For this review, take the finished solid that the model builds, in its own axes (mm). A direction names the side the tool comes from. Round coordinates to 2 decimals unless told otherwise and drop trailing zeros. Order: outer loops, then holes, each group sorted by start corner. A loop starts at its lowest first (then second) coordinate and runs counter-clockwise, first axis right, second up. Notation, with made-up numbers: (-27.5, 24.5) -> (-18.5, 24.5) arc R26 ccw to (-18.5, 43.5) -> close; hole circle Ø1 at (64, 47). An arc over 180 degrees is marked (long way). Use a Markdown table: item, result. Add a question column.
1) Wall thickness on line 1 along Z through (x, y) = (-2.75, -43.8); line 2 along Z through (x, y) = (-6.5, -43.8); line 3 along Z through (x, y) = (-1.75, 55): over which ranges is each line inside the solid? List them lowest first. Write a range as [from, to].
2) Machinability: for faces 5 (the face through (2, -68.8, 0)), 6 (the face through (1.5, -62.37, 16.52)), 7 (the face through (5, 70, 0)), which of the approach directions +Z, -Z, +X, -X, +Y, -Y give a long, thin tool a straight path to every point of the face, cutting with its end or side? Answer none if there is none.
3) Consider section A-A (y = 43.8). State the section outline as (x, z) points, plus the area to 4 significant figures.
4) Clearance check with flat-ended pins moving along their axes: P1, Ø6, axis at x = -3.5, z = -2, coming from the +Y side; P2, Ø6.5, axis at y = 46.5, z = -11.5, coming from the +X side; P3, Ø2, axis at y = 49, z = -1, coming from the +X side; P4, Ø11, axis at y = 43.8, z = 14.05, coming from the -X side. State where each tip first meets the part, or that it passes through.
5) Consider section B-B (y = -31.5). State the section outline as (x, z) points, plus the area to 4 significant figures.
6) Consider section C-C (x = 2). State the section outline as (y, z) points, plus the area to 3 significant figures.
7) Consider section D-D (z = -3.5). State the section outline as (x, y) points.
8) Draft analysis for pull direction Z (two halves, no side actions). For faces 1 (the face through (-4, 1, 19.05)), 2 (the face through (-3.57, 67.3, -0.2)), 3 (the face through (-2.46, -43.67, -8.15)), 4 (the face through (1.43, 62.3, -16.52)), state which applies: pulls with the +Z half, pulls with the -Z half, needs draft (parallel to the pull), parting line crosses it, or undercut.
```python
from build123d import *
from build123d.topology import SkipClean

# Parameters (mm, degrees)
BOSS_EXTRUDE1_DEPTH              = 19.05
CUT_EXTRUDE1_DEPTH               = 77.872247918
CUT_EXTRUDE1_DEPTH_BACK          = 5
SKETCH3_W                        = 28.1
SKETCH3_H                        = 137.6
FILLET1_R                        = 5
FILLET2_R                        = 10
TAP_DRILL_FOR_M8X1_25_TAP1_D     = 6.8
TAP_DRILL_FOR_M8X1_25_TAP1_DEPTH = 12
TAP_DRILL_FOR_M8X1_25_TAP1_TIP   = 2.042926105
BOSS_EXTRUDE2_START              = 5
BOSS_EXTRUDE2_DEPTH              = 5


with BuildPart() as part:
    # Sketch1 → Boss-Extrude1 (new, symmetric)
    with BuildSketch(Plane.XY):
        Polygon((0, 63.8), (0, -63.8), (5, -63.8), (5, -73.8), (-10, -73.8), (-10, 73.8), (5, 73.8), (5, 63.8), align=None)
    extrude(amount=BOSS_EXTRUDE1_DEPTH, both=True)

    # Sketch3 → Cut-Extrude1 (cut, two sides: drawn at the far end of the back side and taken through both)
    with BuildSketch(Plane(origin=(0, 0, 0), x_dir=(0, 0, -1), z_dir=(1, 0, 0)).offset(-CUT_EXTRUDE1_DEPTH_BACK)):
        Rectangle(SKETCH3_W, SKETCH3_H)
    extrude(amount=CUT_EXTRUDE1_DEPTH + CUT_EXTRUDE1_DEPTH_BACK, mode=Mode.SUBTRACT)

    # Fillet1
    fillet1_edges = [part.edges().sort_by_distance(p)[0] for p in [
        (0, -63.8, 16.55),
        (0, -63.8, -16.55),
        (0, 63.8, 16.55),
        (0, 63.8, -16.55),
        (-5, -68.8, 0),
        (-5, 68.8, 0),
    ]]
    fillet(fillet1_edges, radius=FILLET1_R - 0.0001)  # a hair under: the kernel refuses the full size

    # Fillet2
    fillet2_edges = [part.edges().sort_by_distance(p)[0] for p in [
        (-10, -73.8, 0),
        (-10, 73.8, 0),
    ]]
    fillet(fillet2_edges, radius=FILLET2_R)

    # Tap Drill for M8x1.25 Tap1
    with Locations(Plane.ZY.offset(10)):
        with Locations((-14.05, 43.8), (14.05, 43.8), (-14.05, -43.8), (14.05, -43.8)):
            Hole(TAP_DRILL_FOR_M8X1_25_TAP1_D / 2, depth=TAP_DRILL_FOR_M8X1_25_TAP1_DEPTH)
            with Locations((0, 0, -(TAP_DRILL_FOR_M8X1_25_TAP1_DEPTH + TAP_DRILL_FOR_M8X1_25_TAP1_TIP / 2))):  # 118° drill point
                Cone(0, TAP_DRILL_FOR_M8X1_25_TAP1_D / 2, TAP_DRILL_FOR_M8X1_25_TAP1_TIP, mode=Mode.SUBTRACT)

    # Sketch6 → Boss-Extrude2 (add)
    with SkipClean():  # the faces are left unmerged after this step: merging them gives an invalid solid
        with BuildSketch(Plane(origin=(-5, 0, 0), x_dir=(0, 0, -1), z_dir=(1, 0, 0)).offset(BOSS_EXTRUDE2_START)):
            with BuildLine():
                Line((14.05, -40.4), (14.05, -37.9))
                ThreePointArc((14.05, -37.9), (8.15, -43.8), (14.05, -49.7))
                Line((14.05, -49.7), (14.05, -47.2))
                ThreePointArc((14.05, -47.2), (10.65, -43.8), (14.05, -40.4))
            make_face()
            with BuildLine():
                ThreePointArc((-14.05, -49.7), (-8.15, -43.8), (-14.05, -37.9))
                Line((-14.05, -37.9), (-14.05, -40.4))
                ThreePointArc((-14.05, -40.4), (-10.65, -43.8), (-14.05, -47.2))
                Line((-14.05, -47.2), (-14.05, -49.7))
            make_face()
            with BuildLine():
                Line((14.05, 47.2), (14.05, 49.7))
                ThreePointArc((14.05, 49.7), (8.15, 43.8), (14.05, 37.9))
                Line((14.05, 37.9), (14.05, 40.4))
                ThreePointArc((14.05, 40.4), (10.65, 43.8), (14.05, 47.2))
            make_face()
            with BuildLine():
                ThreePointArc((-14.05, 49.7), (-8.15, 43.8), (-14.05, 37.9))
                Line((-14.05, 37.9), (-14.05, 40.4))
                ThreePointArc((-14.05, 40.4), (-10.65, 43.8), (-14.05, 47.2))
                Line((-14.05, 47.2), (-14.05, 49.7))
            make_face()
        extrude(amount=-BOSS_EXTRUDE2_DEPTH)


solid = part.part
```
Results list:
| question | item | result |
|---|---|---|
| 1 | line 1 | [-19.05, -17.45], [-10.65, -8.15], [8.15, 10.65], [17.45, 19.05] |
| 1 | line 2 | [-19.05, -17.45], [-10.65, 10.65], [17.45, 19.05] |
| 1 | line 3 | [-19.05, -14.05], [14.05, 19.05] |
| 2 | face 5 | +X |
| 2 | face 6 | +Z, -Z, +X |
| 2 | face 7 | +Z, -Z, +X, +Y, -Y |
| 3 | outline | (-10, -19.05) -> (0, -19.05) -> (0, -17.45) -> (-10, -17.45) -> close; (-10, -10.65) -> (0, -10.65) -> (0, -8.15) -> (-5, -8.15) -> (-5, 8.15) -> (0, 8.15) -> (0, 10.65) -> (-10, 10.65) -> close; (-10, 17.45) -> (0, 17.45) -> (0, 19.05) -> (-10, 19.05) -> close |
| 3 | area | 163.5 mm2 |
| 4 | P1 | y = 73.79 |
| 4 | P2 | x = 0 |
| 4 | P3 | x = -5 |
| 4 | P4 | x = -10 |
| 5 | outline | (-10, -19.05) -> (0, -19.05) -> (0, -14.05) -> (-5, -14.05) -> (-5, 14.05) -> (0, 14.05) -> (0, 19.05) -> (-10, 19.05) -> close |
| 5 | area | 240.5 mm2 |
| 6 | outline | (-73.8, -19.05) -> (-62.8, -19.05) -> (-62.8, -14.05) -> (-68.8, -14.05) -> (-68.8, 14.05) -> (-62.8, 14.05) -> (-62.8, 19.05) -> (-73.8, 19.05) -> close; (62.8, -19.05) -> (73.8, -19.05) -> (73.8, 19.05) -> (62.8, 19.05) -> (62.8, 14.05) -> (68.8, 14.05) -> (68.8, -14.05) -> (62.8, -14.05) -> close |
| 6 | area | 501 mm2 |
| 7 | outline | (-10, -63.8) arc R10 ccw to (0, -73.8) -> (5, -73.8) -> (5, -68.8) -> (0, -68.8) arc R5 cw to (-5, -63.8) -> (-5, 63.8) arc R5 cw to (0, 68.8) -> (5, 68.8) -> (5, 73.8) -> (0, 73.8) arc R10 ccw to (-10, 63.8) -> close |
| 8 | face 1 | pulls with the +Z half |
| 8 | face 2 | undercut |
| 8 | face 3 | undercut |
| 8 | face 4 | needs draft |
